Read the model definition and answer for the solid it produces. Units are mm, in the model's axes. A direction names the side the tool comes from. Give positions to 0.01 mm unless a question says otherwise; leave off trailing zeros. Order: outer loops, then holes, each group sorted by start corner. A loop starts at its lowest first (then second) coordinate and runs counter-clockwise, first axis right, second up. Notation, with made-up numbers: M 16.5,27.5 L 29.5,27.5 A13 ccw 29.5,33.5 Z; hole C 49,3 d7. An arc over 180 degrees is marked long. One line per item, written item: value.
from build123d import *

# Parameters (mm, degrees)
F0_W     = 30
F0_H     = 30
F0_R     = 3.5
F1_DEPTH = 1.5875


# Not quite as in the source:
# - a length typed as a fraction of an inch, garbled in the dataset ("3 / 203.2 mm" for 3/8 in), is restored


with BuildPart() as f1:
    # F0 (on Top) → F1 (new body)
    with BuildSketch(Plane.XY):
        with Locations((-1.1622245609, -0.8481781135)):
            Rectangle(F0_W, F0_H)
        with BuildLine():
            Line((-13.8210662203, -10.8358568401), (-8.2036473316, -5.1398402471))
            ThreePointArc((-8.2036473316, -5.1398402471), (-5.3752884611, -5.120190821), (-5.355639035, -7.9485496914))
            Line((-5.355639035, -7.9485496914), (-10.9730579238, -13.6445662845))
            ThreePointArc((-10.9730579238, -13.6445662845), (-13.8014167942, -13.6642157105), (-13.8210662203, -10.8358568401))
        make_face(mode=Mode.SUBTRACT)
        with BuildLine():
            ThreePointArc((3.0311899132, -7.9485496914), (3.0508393392, -5.120190821), (5.8791982097, -5.1398402471))
            Line((5.8791982097, -5.1398402471), (11.4966170985, -10.8358568401))
            ThreePointArc((11.4966170985, -10.8358568401), (11.4769676724, -13.6642157105), (8.6486088019, -13.6445662845))
            Line((8.6486088019, -13.6445662845), (3.0311899132, -7.9485496914))
        make_face(mode=Mode.SUBTRACT)
        with Locations((-1.1622245609, -0.8481781135)):
            Circle(F0_R, mode=Mode.SUBTRACT)
        with BuildLine():
            ThreePointArc((-5.355639035, 6.2521934645), (-5.3752884611, 3.423834594), (-8.2036473316, 3.4434840201))
            Line((-8.2036473316, 3.4434840201), (-13.8210662203, 9.1395006131))
            ThreePointArc((-13.8210662203, 9.1395006131), (-13.8014167942, 11.9678594836), (-10.9730579238, 11.9482100575))
            Line((-10.9730579238, 11.9482100575), (-5.355639035, 6.2521934645))
        make_face(mode=Mode.SUBTRACT)
        with BuildLine():
            Line((3.0311899132, 6.2521934645), (8.6486088019, 11.9482100575))
            ThreePointArc((8.6486088019, 11.9482100575), (11.4769676724, 11.9678594836), (11.4966170985, 9.1395006131))
            Line((11.4966170985, 9.1395006131), (5.8791982097, 3.4434840201))
            ThreePointArc((5.8791982097, 3.4434840201), (3.0508393392, 3.423834594), (3.0311899132, 6.2521934645))
        make_face(mode=Mode.SUBTRACT)
    extrude(amount=F1_DEPTH)


solid = f1.part
1) Find section C-C, the plane y = -12.5. Write down the section's boundary in (x, z).
Reported:
outline: M -16.16,0 L -14.38,0 L -14.38,1.59 L -16.16,1.59 Z; M -9.84,0 L 7.52,0 L 7.52,1.59 L -9.84,1.59 Z; M 12.06,0 L 13.84,0 L 13.84,1.59 L 12.06,1.59 Z
2) Find section A-A, the plane x = -10. Write down the section's boundary in (y, z).
Reported:
outline: M -15.85,0 L -12.66,0 L -12.66,1.59 L -15.85,1.59 Z; M -6.96,0 L 5.26,0 L 5.26,1.59 L -6.96,1.59 Z; M 10.96,0 L 14.15,0 L 14.15,1.59 L 10.96,1.59 Z
3) Which of the six approach directions +Z, -Z, +X, -X, +Y, -Y give full straight-line access (tool end or side, diameter ignored) to faces 1 (the face through (-1, -15.848, 1)), 2 (the face through (8.727, 6.331, 0.783))?
Reported:
face 1: +Z, -Z, +X, -X, -Y
face 2: +Z, -Z
4) Find section B-B, the plane y = 1.75. Write down the section's boundary in (x, z).
Reported:
outline: M -16.16,0 L -3.51,0 L -3.51,1.59 L -16.16,1.59 Z; M 1.18,0 L 13.84,0 L 13.84,1.59 L 1.18,1.59 Z
5) Determine the mould class of faces 3 (the face through (8.6, -7.9, 0.8)), 4 (the face through (-1, 3, 0)), 5 (the face through (-16.162, -1, 1)) for opening direction X: +X half, -X half, draft (parallel to the pull), parting line (faces both ways), or undercut.
Reported:
face 3: undercut
face 4: draft
face 5: -X half
6) Find section D-D, the plane x = -4.25. Write down the section's boundary in (y, z).
Reported:
outline: M -15.85,0 L -2.5,0 L -2.5,1.59 L -15.85,1.59 Z; M 0.8,0 L 14.15,0 L 14.15,1.59 L 0.8,1.59 Z
7) Consider probe 1 along X at (y, z) = (4.25, 0.7); probe 2 along X at (y, z) = (-5.5, 1.2); probe 3 along Y at (x, z) = (-7, 0.2). Determine where each line is inside the solid, lowest interval first.
Reported:
probe 1: x = -16.16 to -9, -4.87 to 2.55, 6.67 to 13.84
probe 2: x = -16.16 to -8.56, -5.07 to 2.75, 6.23 to 13.84
probe 3: y = -15.85 to -9.62, -4.56 to 2.86, 7.92 to 14.15
